```python
from build123d import *

# Parameters (mm, degrees)
BOSS_EXTRUDE1_DEPTH = 3.175
FILLET1_R           = 5
SKETCH2_R           = 1.6
CUT_EXTRUDE1_DEPTH  = 4.175


with BuildPart() as part:
    # Sketch1 → Boss-Extrude1 (new body)
    with BuildSketch(Plane.XY):
        Polygon((0, 54), (0, 0), (30, 0), (30, 15), (15, 15), (15, 39), (30, 39), (30, 54), align=None)
    extrude(amount=BOSS_EXTRUDE1_DEPTH)

    # Fillet1
    fillet1_edges = [part.edges().sort_by_distance(p)[0] for p in [
        (15, 15, 1.5875),
        (30, 15, 1.5875),
        (30, 0, 1.5875),
        (0, 0, 1.5875),
        (0, 54, 1.5875),
        (30, 54, 1.5875),
        (30, 39, 1.5875),
        (15, 39, 1.5875),
    ]]
    fillet(fillet1_edges, radius=FILLET1_R)

    # Sketch2 → Cut-Extrude1 (cut, through all)
    with BuildSketch(Plane.XY.offset(3.175)):
        with Locations((7.5, 7.5)):
            Circle(SKETCH2_R)
        with Locations((7.5, 46.5)):
            Circle(SKETCH2_R)
        with Locations((22.5, 7.5)):
            Circle(SKETCH2_R)
        with Locations((7.5, 27)):
            Circle(SKETCH2_R)
        with Locations((22.5, 46.5)):
            Circle(SKETCH2_R)
    extrude(amount=-CUT_EXTRUDE1_DEPTH, mode=Mode.SUBTRACT)


solid = part.part
```
Source: CAD feature listing. Evaluate the final solid. Frame: model axes, mm. A direction names the side the tool comes from. Coordinates: 2 decimals unless noted, no trailing zeros. Loops run counter-clockwise (first coordinate to the right, second up) from the corner with the lowest first, then second, coordinate; pieces in that order, holes last. Notation, with made-up numbers: (67.25, 58) - (115.25, 58) arc R29 cw to (115.25, 96) - close; hole circle Ø7 at (20.25, -28). An arc over 180 degrees is marked (long way). Answer as CSV lines item,"result".
1. Section D-D (z = 2.5). Return loops of the section in (x, y), then the cut area to 3 significant figures.
Established:
outline,"(0, 5) arc R5 ccw to (5, 0) - (25, 0) arc R5 ccw to (30, 5) - (30, 10) arc R5 ccw to (25, 15) - (20, 15) arc R5 cw to (15, 20) - (15, 34) arc R5 cw to (20, 39) - (25, 39) arc R5 ccw to (30, 44) - (30, 49) arc R5 ccw to (25, 54) - (5, 54) arc R5 ccw to (0, 49) - close; hole circle Ø3.2 at (7.5, 7.5); hole circle Ø3.2 at (7.5, 27); hole circle Ø3.2 at (7.5, 46.5); hole circle Ø3.2 at (22.5, 7.5); hole circle Ø3.2 at (22.5, 46.5)"
area,"1,200 mm2"
2. Ray query, line 1 (Y direction, x = 22.5, z = 1.3); line 2 (Y direction, x = 7.5, z = 1.25); line 3 (X direction, y = 22.5, z = 1.1). Return the intervals inside material, ascending.
Established:
line 1,"y = 0 to 5.9, 9.1 to 15, 39 to 44.9, 48.1 to 54"
line 2,"y = 0 to 5.9, 9.1 to 25.4, 28.6 to 44.9, 48.1 to 54"
line 3,"x = 0 to 15"
3. Section B-B (y = 27). Return loops of the section in (x, z) (3 decimals).
Established:
outline,"(0, 0) - (5.9, 0) - (5.9, 3.175) - (0, 3.175) - close; (9.1, 0) - (15, 0) - (15, 3.175) - (9.1, 3.175) - close"
4. Mould query, pull axis Y, two halves, no side actions, for faces 1 (the cylindrical face through (1, 2, 2)), 2 (the cylindrical face through (16, 37, 2)), 3 (the flat face through (30, 46, 2)). Classes: released by +Y, released by -Y, zero draft, split by the parting line, or undercut.
Established:
face 1,"released by -Y"
face 2,"undercut"
face 3,"zero draft"
5. Section C-C (y = 7.5). Return loops of the section in (x, z) (3 decimals).
Established:
outline,"(0, 0) - (5.9, 0) - (5.9, 3.175) - (0, 3.175) - close; (9.1, 0) - (20.9, 0) - (20.9, 3.175) - (9.1, 3.175) - close; (24.1, 0) - (30, 0) - (30, 3.175) - (24.1, 3.175) - close"
6. Contact query for flat-ended pins moving along their axis: pin 1 (10 mm diameter, centred on x = 21, y = 29, fed in from -Z); pin 2 (4 mm diameter, centred on x = 22.5, y = 46.5, fed in from +Z) (3 decimals); pin 3 (1 mm diameter, centred on y = 29.5, z = 2, fed in from +X). Output: stop coordinate, or through.
Established:
pin 1,"passes through"
pin 2,"stops at z = 3.175"
pin 3,"stops at x = 15"
7. Reachability of faces 4 (the cylindrical face through (17, 16, 2)), 5 (the cylindrical face through (1, 52, 2)) from +Z, -Z, +X, -X, +Y, -Y: full face, straight path, thin tool, end or side. Return the list, or none.
Established:
face 4,"+Z, -Z, +X"
face 5,"+Z, -Z, -X, +Y"
8. Section A-A (x = 7.5). Return loops of the section in (y, z) (3 decimals).
Established:
outline,"(0, 0) - (5.9, 0) - (5.9, 3.175) - (0, 3.175) - close; (9.1, 0) - (25.4, 0) - (25.4, 3.175) - (9.1, 3.175) - close; (28.6, 0) - (44.9, 0) - (44.9, 3.175) - (28.6, 3.175) - close; (48.1, 0) - (54, 0) - (54, 3.175) - (48.1, 3.175) - close"
